Work out the finished part from the listing and answer in its coordinate system (mm). A direction names the side the tool comes from. Round coordinates to 2 decimals unless told otherwise and drop trailing zeros. Write each loop counter-clockwise with the first axis right and the second up, starting at its lowest first coordinate (ties: lowest second). Pieces come first, ordered by that corner, then holes.
1. Flat-ended cylindrical pins translate along their axes: pin 1 Ø4 at (x, z) = (-27.5, 21.5) entering from +Y; pin 2 Ø1.6 at (x, z) = (3, 25) entering from +Y; pin 3 Ø3 at (x, y) = (-3.5, -84.5) entering from -Z; pin 4 Ø18 at (y, z) = (-89.61, 16) entering from +X. Find the tip coordinate at first contact, or state that the pin passes through.
2. Find section B-B (x = -32). Write down the section's boundary in (y, z).
3. Determine the mould class of faces 1 (the face through (-10, -91, 0)), 2 (the face through (-4, -67.792, 46)), 3 (the face through (-39, -114, 44)) for opening direction X: pulls with the +X half, pulls with the -X half, needs draft (parallel to the pull), parting line crosses it, or undercut.
4. A tool of negligible diameter and unlimited length cuts with its end or side. For faces 4 (the face through (-10, -69.792, 46)), 5 (the face through (-10, -116, 44)), 6 (the face through (2, -102, 37)), from which of +Z, -Z, +X, -X, +Y, -Y can it reach the whole face along a straight path? Write none if from no direction.
5. Straight lines are drawn through the part: probe 1 along Y at (x, z) = (-16.5, 79.5); probe 2 along X at (y, z) = (-111, 60); probe 3 along Y at (x, z) = (-32, 74). For each, find the intervals that lie inside material, in ascending order.
6. Find section A-A (y = -93.5). Write down the section's boundary in (x, z), and give its area (3 significant figures).
```python
from build123d import *

# Parameters (mm, degrees)
F1_DEPTH  = 90
F2_T      = -2
F4_DEPTH  = 90
F5_R      = 5
F6_DEPTH  = 25
F7_W      = 10.9698139131
F7_H      = 3
F7_W_2    = 3
F7_H_2    = 5
F8_DEPTH  = 10
F10_DEPTH = 70
F11_R     = 10
F12_DEPTH = 20
F13_R     = 5
F14_SIZE2 = 5
F14_SIZE  = 2
F15_R     = 1
F16_R     = 2.95
F17_DEPTH = 25


# Not quite as in the source:
# - a feature names something its author has since deleted; it is built from what else it names


with BuildPart() as f1:
    # F0 (on Top) → F1 (new body)
    with BuildSketch(Plane.XY):
        with BuildLine():
            Line((-35, -116), (0, -116))
            Line((0, -116), (15, -116))
            ThreePointArc((15, -116), (18.5355339059, -114.5355339059), (20, -111))
            Line((20, -111), (20, -76))
            ThreePointArc((20, -76), (18.5355339059, -72.4644660941), (15, -71))
            Line((15, -71), (-35, -71))
            ThreePointArc((-35, -71), (-38.5355339059, -72.4644660941), (-40, -76))
            Line((-40, -76), (-40, -111))
            ThreePointArc((-40, -111), (-38.5355339059, -114.5355339059), (-35, -116))
        make_face()
    extrude(amount=F1_DEPTH)

    # F2
    f2_openings = [f1.faces().sort_by_distance(p)[0] for p in [
        (-10, -93.5, 90),
    ]]
    offset(amount=F2_T, openings=f2_openings)

    # F3 (on face) → F4 (join, through all)
    with BuildSketch(Plane.XY.offset(90)):
        Polygon((-20, -65.7917543815), (-20, -71), (-10, -71), (0, -71), (0, -65.7917543815), (-5.9066830128, -65.7917543815), (-5.9066830128, -67.7917543815), (-2, -67.7917543815), (-2, -69.7917543815), (-18, -69.7917543815), (-18, -67.7917543815), (-14.0933169872, -67.7917543815), (-14.0933169872, -65.7917543815), align=None)
    extrude(amount=-F4_DEPTH)

    # F5 (on face) → F6 (cut)
    with BuildSketch(Plane.XZ.offset(116)):
        with Locations((-5, 55)):
            Circle(F5_R)
    extrude(amount=-F6_DEPTH, mode=Mode.SUBTRACT)

    # F7 (on face) → F8 (join)
    with BuildSketch(Plane.XY.offset(2)):
        with Locations((-16.3644514978, -74.5)):
            Rectangle(F7_W, F7_H)
        with Locations((8.5, -78.5)):
            Rectangle(F7_W_2, F7_H_2)
        with Locations((8.5, -98.5)):
            Rectangle(F7_W_2, F7_H_2)
    extrude(amount=F8_DEPTH)

    # F9 (on face) → F10 (join)
    with BuildSketch(Plane.XY.offset(2)):
        Polygon((-34, -101), (-38, -101), (-38, -107), (-34, -107), (-34, -105), (-36, -105), (-36, -103), (-34, -103), align=None)
        Polygon((7, -101), (2, -101), (2, -103), (4, -103), (4, -105), (2, -105), (2, -107), (7, -107), (7, -114), (10, -114), (10, -107), (10, -101), align=None)
    extrude(amount=F10_DEPTH)

    # F11 (on face) → F12 (cut)
    with BuildSketch(Plane.YZ.offset(20)):
        with Locations((-89.6050930023, 72)):
            Circle(F11_R)
        with Locations((-89.6050930023, 44)):
            Circle(F11_R)
        with Locations((-89.6050930023, 16)):
            Circle(F11_R)
    extrude(amount=-F12_DEPTH, mode=Mode.SUBTRACT)

    # F13
    f13_edges = [f1.edges().sort_by_distance(p)[0] for p in [
        (0, -71, 45),
        (-20, -71, 45),
    ]]
    fillet(f13_edges, radius=F13_R)

    # F14
    f14_edges = [f1.edges().sort_by_distance(p)[0] for p in [
        (-16.364451, -76, 12),
    ]]
    f14_side = f1.faces().sort_by_distance((-16.364451, -74.5, 12))[0]
    chamfer(f14_edges, length=F14_SIZE, length2=F14_SIZE2, reference=f14_side)

    # F15
    f15_edges = [f1.edges().sort_by_distance(p)[0] for p in [
        (8.5, -80.439942, 12),
        (8.5, -76, 12),
        (8.5, -98.770244, 12),
        (8.5, -96, 8.312012),
    ]]
    fillet(f15_edges, radius=F15_R)

    # F16 (on face) → F17 (cut)
    with BuildSketch(Plane(origin=(-40, 0, 0), x_dir=(0, -1, 0), z_dir=(-1, 0, 0))):
        with Locations((93.5, 78)):
            Circle(F16_R)
    extrude(amount=-F17_DEPTH, mode=Mode.SUBTRACT)


solid = f1.part
```
Worked answers:
1. pin 1: stops at y = -71
1. pin 2: stops at y = -70.14
1. pin 3: stops at z = 0
1. pin 4: stops at x = -38
2. outline: (-116, 0) - (-71, 0) - (-71, 90) - (-73, 90) - (-73, 2) - (-114, 2) - (-114, 90) - (-116, 90) - close
3. face 1: needs draft
3. face 2: undercut
3. face 3: pulls with the -X half
4. face 4: +Z, -Z
4. face 5: +Z, -Z, +X, -X, -Y
4. face 6: +Z
5. probe 1: y = -116 to -114, -73 to -69.79, -67.79 to -65.79
5. probe 2: x = -40 to -38, 7 to 10, 18 to 20
5. probe 3: y = -116 to -114, -73 to -71
6. outline: (-40, 0) - (20, 0) - (20, 6.79) - (18, 6.79) - (18, 2) - (-38, 2) - (-38, 75.05) - (-40, 75.05) - close; (-40, 80.95) - (-38, 80.95) - (-38, 90) - (-40, 90) - close; (18, 25.21) - (20, 25.21) - (20, 34.79) - (18, 34.79) - close; (18, 53.21) - (20, 53.21) - (20, 62.79) - (18, 62.79) - close; (18, 81.21) - (20, 81.21) - (20, 90) - (18, 90) - close
6. area: 350 mm2
